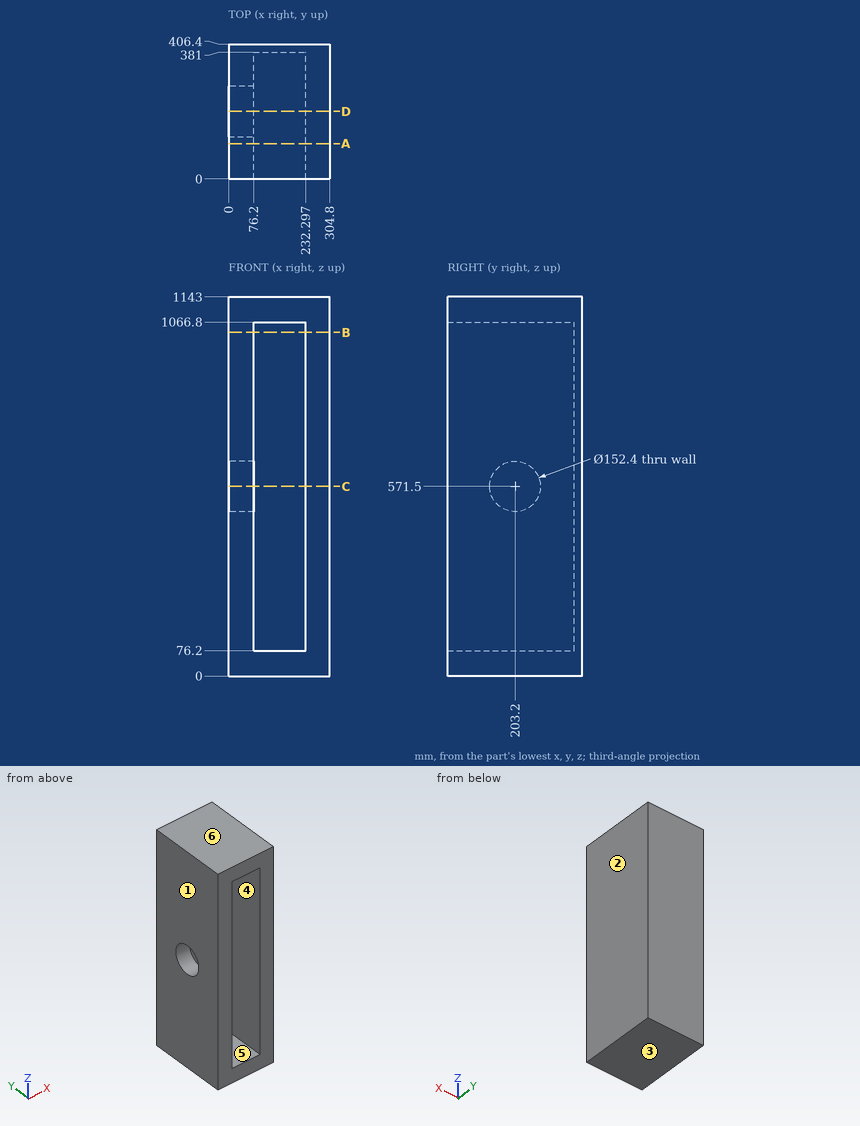
Could you check a few things on this drawing? It's one solid part, dimensions in mm from its lowest x, y, z. A direction names the side the tool comes from. Give positions to 0.01 mm unless a question says otherwise; leave off trailing zeros. Order: outer loops, then holes, each group sorted by start corner. A loop starts at its lowest first (then second) coordinate and runs counter-clockwise, first axis right, second up. Notation, with made-up numbers: (63, 59) - (78, 59) arc R15 cw to (78, 66) - close; hole circle Ø6 at (54, 49.25). An arc over 180 degrees is marked (long way). One line per item, written item: value. Start each with the question number.
1. Thinking about a two-plate mould opening in X: for the marked faces 1, 2, 3 and 4, which applies, +X half, -X half, draft (parallel to the pull), parting line (faces both ways), or undercut?
2. Imagine slicing it at C-C on z = 571.5. List the corners of the cut face in (x, y) for me.
3. If I drill on probe 1 along Z at (x, y) = (47.5, 203.2); probe 2 along X at (y, z) = (77, 332.5); probe 3 along Y at (x, z) = (45, 571), over which ranges is the centre line in solid material (lowest first)?
4. Imagine slicing it at D-D on y = 203.2. List the corners of the cut face in (x, z) for me.
5. For the marked faces 5 and 6, which set-ups out of +Z, -Z, +X, -X, +Y, -Y let a thin tool reach every point of the face, with its end or its side?
6. Imagine slicing it at B-B on z = 1035.5. List the corners of the cut face in (x, y) for me, plus the area to 3 significant figures.
7. Imagine slicing it at A-A on y = 106. List the corners of the cut face in (x, z) for me, plus the area to 3 significant figures.
Values:
1. face 1: -X half
1. face 2: +X half
1. face 3: draft
1. face 4: undercut
2. outline: (0, 0) - (76.2, 0) - (76.2, 127) - (0, 127) - close; (0, 279.4) - (76.2, 279.4) - (76.2, 381) - (232.3, 381) - (232.3, 0) - (304.8, 0) - (304.8, 406.4) - (0, 406.4) - close
3. probe 1: 0 to 495.3, 647.7 to 1143
3. probe 2: 0 to 76.2, 232.3 to 304.8
3. probe 3: 0 to 127, 279.4 to 406.4
4. outline: (0, 0) - (304.8, 0) - (304.8, 1143) - (0, 1143) - (0, 647.7) - (76.2, 647.7) - (76.2, 1066.8) - (232.3, 1066.8) - (232.3, 76.2) - (76.2, 76.2) - (76.2, 495.3) - (0, 495.3) - close
5. face 5: -Y
5. face 6: +Z, +X, -X, +Y, -Y
6. outline: (0, 0) - (76.2, 0) - (76.2, 381) - (232.3, 381) - (232.3, 0) - (304.8, 0) - (304.8, 406.4) - (0, 406.4) - close
6. area: 64,400 mm²
7. outline: (0, 0) - (304.8, 0) - (304.8, 1143) - (0, 1143) - close; hole (76.2, 76.2) - (232.3, 76.2) - (232.3, 1066.8) - (76.2, 1066.8) - close
7. area: 194,000 mm²
